Could you check a few things on this drawing? It's one solid part, dimensions in mm from its lowest x, y, z. A direction names the side the tool comes from. Round coordinates to 2 decimals unless told otherwise and drop trailing zeros. Loops run counter-clockwise (first coordinate to the right, second up) from the corner with the lowest first, then second, coordinate; pieces in that order, holes last. Notation, with made-up numbers: M 22.5,14 L 69.5,14 A22 cw 69.5,34 Z; hole C -22,48.5 d10. An arc over 180 degrees is marked long. Answer as CSV lines item,"result".
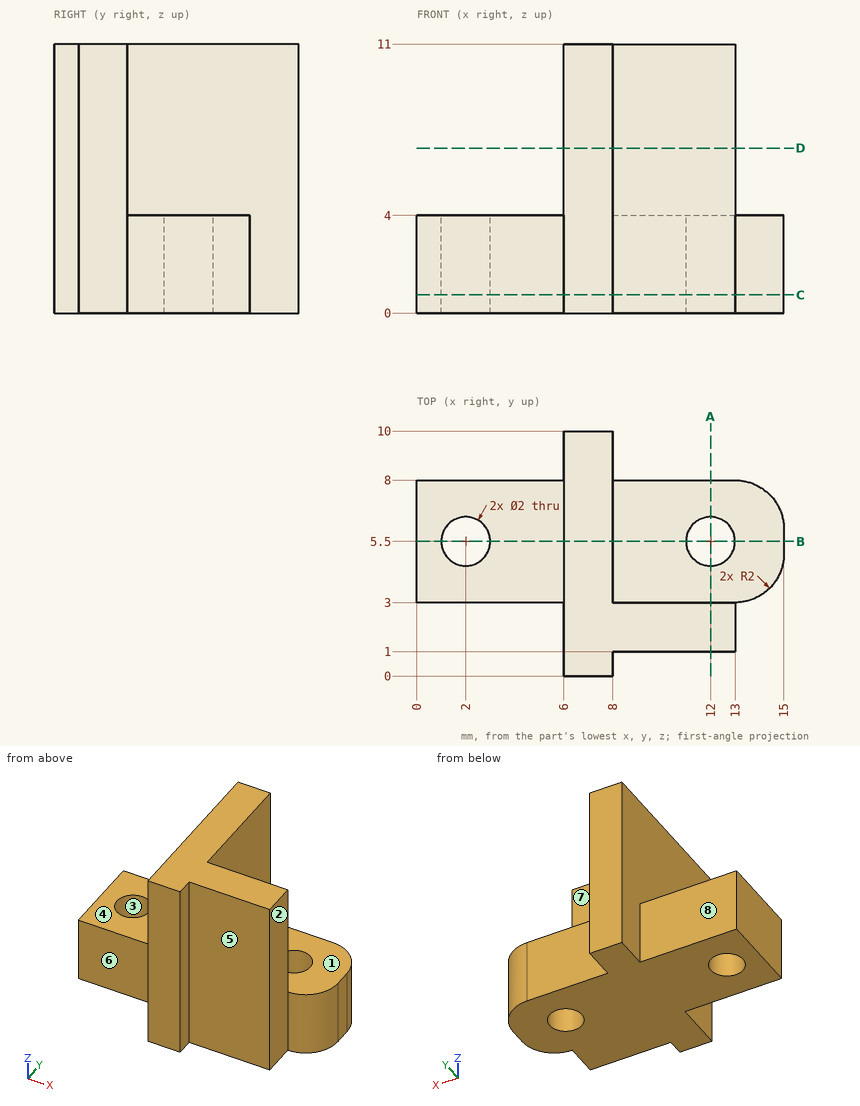
Item 1: On a 3-axis mill with a long thin cutter (end or side, diameter ignored), from which of +Z, -Z, +X, -X, +Y, -Y can I reach the whole of each face in a straight line? I mean the marked faces 4, 5, 6, 7 and 8. Say none if no direction works.
Output:
face 4,"+Z, -X, +Y, -Y"
face 5,"+Z, -Z, +X, -Y"
face 6,"+Z, -Z, -X, -Y"
face 7,"+Z, +X, +Y"
face 8,"+Z, -Z, -X, +Y"
Item 2: If we section it at A-A on x = 12: Write out the boundary of the cut face in (y, z), then the cut area to 3 significant figures.
Output:
outline,"M 1,0 L 4.5,0 L 4.5,4 L 3,4 L 3,11 L 1,11 Z; M 6.5,0 L 8,0 L 8,4 L 6.5,4 Z"
area,"34.0 mm2"
Item 3: If we section it at B-B on y = 5.5: Write out the boundary of the cut face in (x, z).
Output:
outline,"M 0,0 L 1,0 L 1,4 L 0,4 Z; M 3,0 L 11,0 L 11,4 L 8,4 L 8,11 L 6,11 L 6,4 L 3,4 Z; M 13,0 L 15,0 L 15,4 L 13,4 Z"
Item 4: If I drill on line 1 along X through (y, z) = (5.5, 1.4); line 2 along X through (y, z) = (4.75, 3.25); line 3 along X through (y, z) = (5.25, 7.25), over which ranges is the centre line in solid material (lowest first)? Write a range as from..to.
Output:
line 1,"x = 0..1, 3..11, 13..15"
line 2,"x = 0..1.34, 2.66..11.34, 12.66..14.98"
line 3,"x = 6..8"
Item 5: If we section it at D-D on z = 6.75: Write out the boundary of the cut face in (x, y), then the cut area to 3 significant figures.
Output:
outline,"M 6,0 L 8,0 L 8,1 L 13,1 L 13,3 L 8,3 L 8,10 L 6,10 Z"
area,"30.0 mm2"
Item 6: We'd pull the mould along X, two halves only. Please class the marked faces 1, 2 and 3: released by +X, released by -X, zero draft, split by the parting line, or undercut.
Output:
face 1,"zero draft"
face 2,"released by +X"
face 3,"undercut"
Item 7: Will these pins go through, and if not, where does the flat tip stop? pin 1 (1.5 mm diameter, centred on x = 4, z = 8, fed in from -Y); pin 2 (2.5 mm diameter, centred on x = 2, y = 5.5, fed in from +Z); pin 3 (4.5 mm diameter, centred on x = 11, z = 1.5, fed in from +Y); pin 4 (0.6 mm diameter, centred on y = 2, z = 4, fed in from +X).
Output:
pin 1,"passes through"
pin 2,"stops at z = 4"
pin 3,"stops at y = 8"
pin 4,"stops at x = 13"
Item 8: If we section it at C-C on z = 0.75: Write out the boundary of the cut face in (x, y).
Output:
outline,"M 0,3 L 6,3 L 6,0 L 8,0 L 8,1 L 13,1 L 13,3 A2 ccw 15,5 L 15,6 A2 ccw 13,8 L 8,8 L 8,10 L 6,10 L 6,8 L 0,8 Z; hole C 2,5.5 d2; hole C 12,5.5 d2"
